```python
from build123d import *

# Parameters (mm, degrees)
BOSS_EXTRUDE1_DEPTH = 3
SKETCH2_W           = 3
SKETCH2_H           = 10
CUT_EXTRUDE1_DEPTH  = 10


with BuildPart() as part:
    # Sketch1 → Boss-Extrude1 (new body)
    with BuildSketch(Plane.XY):
        with BuildLine():
            Line((-5, -21.5), (5, -21.5))
            ThreePointArc((5, -21.5), (13.485281374, -25.014718626), (17, -33.5))
            Line((17, -33.5), (17, -61.5))
            ThreePointArc((17, -61.5), (14.071067812, -68.571067812), (7, -71.5))
            Line((7, -71.5), (0.5, -71.5))
            Line((0.5, -71.5), (-0.5, -71.5))
            Line((-0.5, -71.5), (-7, -71.5))
            ThreePointArc((-7, -71.5), (-14.071067812, -68.571067812), (-17, -61.5))
            Line((-17, -61.5), (-17, -33.5))
            ThreePointArc((-17, -33.5), (-13.485281374, -25.014718626), (-5, -21.5))
        make_face()
    extrude(amount=BOSS_EXTRUDE1_DEPTH)

    # Sketch2 → Cut-Extrude1 (cut)
    with BuildSketch(Plane.XY.offset(3)):
        with Locations((0, -48)):
            Rectangle(SKETCH2_W, SKETCH2_H)
    extrude(amount=-CUT_EXTRUDE1_DEPTH, mode=Mode.SUBTRACT)


solid = part.part
```
Could you check a few things on this model? Use its own coordinates, in mm. A direction names the side the tool comes from. Give positions to 0.01 mm unless a question says otherwise; leave off trailing zeros. Order: outer loops, then holes, each group sorted by start corner. A loop starts at its lowest first (then second) coordinate and runs counter-clockwise, first axis right, second up.
Q1. For faces 1 (the flat face through (-17, -48, 1)), 2 (the flat face through (-1.5, -48, 2)), which set-ups out of +Z, -Z, +X, -X, +Y, -Y let a thin tool reach every point of the face, with its end or its side?
Q2. We'd pull the mould along X, two halves only. Please class faces 3 (the cylindrical face through (-13.58, -25.11, 1.48)), 4 (the cylindrical face through (14.15, -68.49, 1.48)), 5 (the flat face through (0, -43, 2)): +X half, -X half, draft (parallel to the pull), parting line (faces both ways), or undercut.
Q3. Suppose I cut it at A-A, the plane x = 0. Write out the boundary of the cut face in (y, z), and give its area (3 significant figures).
Q4. Suppose I cut it at B-B, the plane z = 2.5. Write out the boundary of the cut face in (x, y).
Q5. Suppose I cut it at D-D, the plane y = -29. Write out the boundary of the cut face in (x, z), and give its area (3 significant figures).
Q6. If I drill on line 1 along X through (y, z) = (-52, 2.6); line 2 along Y through (x, z) = (-9, 2.3); line 3 along X through (y, z) = (-68, 0.3), over which ranges is the centre line in solid material (lowest first)?
Q7. Suppose I cut it at C-C, the plane y = -43.5. Write out the boundary of the cut face in (x, z), and give its area (3 significant figures).
Solution:
1. face 1: +Z, -Z, -X, +Y, -Y
1. face 2: +Z, -Z
2. face 3: -X half
2. face 4: +X half
2. face 5: undercut
3. outline: (-71.5, 0) - (-53, 0) - (-53, 3) - (-71.5, 3) - close; (-43, 0) - (-21.5, 0) - (-21.5, 3) - (-43, 3) - close
3. area: 120 mm2
4. outline: (-17, -61.5) arc R10 ccw to (-7, -71.5) - (7, -71.5) arc R10 ccw to (17, -61.5) - (17, -33.5) arc R12 ccw to (5, -21.5) - (-5, -21.5) arc R12 ccw to (-17, -33.5) - close; hole (-1.5, -53) - (1.5, -53) - (1.5, -43) - (-1.5, -43) - close
5. outline: (-16.12, 0) - (16.12, 0) - (16.12, 3) - (-16.12, 3) - close
5. area: 96.7 mm2
6. line 1: x = -17 to -1.5, 1.5 to 17
6. line 2: y = -71.3 to -22.19
6. line 3: x = -14.6 to 14.6
7. outline: (-17, 0) - (-1.5, 0) - (-1.5, 3) - (-17, 3) - close; (1.5, 0) - (17, 0) - (17, 3) - (1.5, 3) - close
7. area: 93.0 mm2
